For this review, take the finished solid that the model builds, in its own axes (mm). A direction names the side the tool comes from. Round coordinates to 2 decimals unless told otherwise and drop trailing zeros. Order: outer loops, then holes, each group sorted by start corner. A loop starts at its lowest first (then second) coordinate and runs counter-clockwise, first axis right, second up. Notation, with made-up numbers: (12, -28.75) - (41, -28.75) arc R24 ccw to (41, 1.25) - close; hole circle Ø3 at (-24, -31.75). An arc over 180 degrees is marked (long way). Write each question's results on one line, items separated by ' | '. Start each with the question number.
(1) Take a section at A-A, the plane x = 19.05. Give the boundary of the cut face in (y, z) (3 decimals).
(2) For L1, parallel to Y at x = 19.05, z = 0.7; L2, parallel to Y at x = 29.5, z = 2.1; L3, parallel to X at y = 5.5, z = 1.6 (3 decimals), list the stretches that pass through material, from the lowest coordinate up. Write a range as from..to.
(3) Take a section at C-C, the plane y = 2.25. Give the boundary of the cut face in (x, z) (1 decimal), plus the area to 3 significant figures.
(4) For faces 1 (the flat face through (14.288, 3, 2)), 2 (the flat face through (2, 7.938, 2)), 3 (the flat face through (36, 7.938, 2)), list the 3-axis set-ups (+Z, -Z, +X, -X, +Y, -Y) from which the entire face can be reached by the end or side of a thin tool; tool diameter is ignored.
(5) Take a section at D-D, the plane y = 12.7. Give the boundary of the cut face in (x, z) (3 decimals).
(6) Draft analysis for pull direction X (two halves, no side actions). For faces 4 (the flat face through (19, 25.4, 2)), 5 (the cylindrical face through (17.3, 3.3, 1.6)), 6 (the flat face through (3.175, 6, 2)), state which applies: pulls with the +X half, pulls with the -X half, needs draft (parallel to the pull), parting line crosses it, or undercut.
(7) Insertion check: pin 1 Ø1.7 at (y, z) = (0.5, 1) entering from -X (3 decimals); pin 2 Ø1 at (x, z) = (1.5, 1.5) entering from -Y; pin 3 Ø3 at (x, y) = (1.42, 12.7) entering from +Z; pin 4 Ø1.6 at (y, z) = (3.5, 2) entering from -X. Each pin has a flat end and moves straight along its axis. Give the tip position at first contact, or say it passes through.
```python
from build123d import *

# Parameters (mm, degrees)
SKETCH1_R           = 1.7526
BOSS_EXTRUDE1_DEPTH = 3.175


with BuildPart() as part:
    # Sketch1 → Boss-Extrude1 (new body)
    with BuildSketch(Plane.XY):
        with BuildLine():
            Line((3.175, 1.5875), (3.175, 0))
            Line((3.175, 0), (34.925, 0))
            Line((34.925, 0), (34.925, 1.5875))
            Line((34.925, 1.5875), (23.8125, 1.5875))
            Line((23.8125, 1.5875), (23.8125, 4.7625))
            Line((23.8125, 4.7625), (34.925, 4.7625))
            Line((34.925, 4.7625), (34.925, 7.9375))
            Line((34.925, 7.9375), (38.1, 7.9375))
            Line((38.1, 7.9375), (38.1, 11.676093266))
            ThreePointArc((38.1, 11.676093266), (34.925, 12.7), (38.1, 13.723906734))
            Line((38.1, 13.723906734), (38.1, 17.4625))
            Line((38.1, 17.4625), (34.925, 17.4625))
            Line((34.925, 17.4625), (34.925, 25.4))
            Line((34.925, 25.4), (3.175, 25.4))
            Line((3.175, 25.4), (3.175, 17.4625))
            Line((3.175, 17.4625), (0, 17.4625))
            Line((0, 17.4625), (0, 13.723906734))
            ThreePointArc((0, 13.723906734), (3.175, 12.7), (0, 11.676093266))
            Line((0, 11.676093266), (0, 7.9375))
            Line((0, 7.9375), (3.175, 7.9375))
            Line((3.175, 7.9375), (3.175, 4.7625))
            Line((3.175, 4.7625), (14.2875, 4.7625))
            Line((14.2875, 4.7625), (14.2875, 1.5875))
            Line((14.2875, 1.5875), (3.175, 1.5875))
        make_face()
        with Locations((19.05, 3.175)):
            Circle(SKETCH1_R, mode=Mode.SUBTRACT)
    extrude(amount=BOSS_EXTRUDE1_DEPTH)


solid = part.part
```
Results below:
1) outline: (0, 0) - (1.422, 0) - (1.422, 3.175) - (0, 3.175) - close; (4.928, 0) - (25.4, 0) - (25.4, 3.175) - (4.928, 3.175) - close
2) L1: y = 0..1.42, 4.93..25.4 | L2: y = 0..1.59, 4.76..25.4 | L3: x = 3.175..34.925
3) outline: (14.3, 0) - (17.6, 0) - (17.6, 3.2) - (14.3, 3.2) - close; (20.5, 0) - (23.8, 0) - (23.8, 3.2) - (20.5, 3.2) - close | area: 20.8 mm^2
4) face 1: +Z, -Z, -X | face 2: +Z, -Z, -X, -Y | face 3: +Z, -Z, +X, -Y
5) outline: (3.175, 0) - (34.925, 0) - (34.925, 3.175) - (3.175, 3.175) - close
6) face 4: needs draft | face 5: undercut | face 6: pulls with the -X half
7) pin 1: stops at x = 3.175 | pin 2: stops at y = 7.94 | pin 3: passes through | pin 4: stops at x = 14.29
